from build123d import *

# Parameters (mm, degrees)
F1_DEPTH  = 38
F3_DEPTH  = 25
F4_DEPTH  = 38
F0_W      = 5
F0_H      = 28
F5_DEPTH  = 38
F6_DEPTH  = 34
F0_W_2    = 8.5
F0_H_2    = 23
F7_DEPTH  = 29
F8_DEPTH  = 24
F0_W_3    = 25
F9_DEPTH  = 19
F10_DEPTH = 10
F0_H_3    = 10
F11_DEPTH = 5
F12_DEPTH = 19


with BuildPart() as f1:
    # F0 (on Top) → F1 (new body)
    with BuildSketch(Plane.XY):
        Polygon((-33.5, -24), (-33.5, -14), (-33.5, -4), (-33.5, 19), (-38.5, 19), (-38.5, -24), align=None)
    extrude(amount=F1_DEPTH)

    # F2 (on face) → F3 (cut)
    with BuildSketch(Plane.YZ.offset(-33.5)):
        Polygon((-24, 19), (19, 38), (-24, 38), align=None)
    extrude(amount=-F3_DEPTH, mode=Mode.SUBTRACT)

    # F0 (on Top) → F4 (join)
    with BuildSketch(Plane.XY):
        Polygon((8.5, 19), (8.5, 24), (-38.5, 24), (-38.5, 19), (-33.5, 19), (-8.5, 19), (0, 19), align=None)
    extrude(amount=F4_DEPTH)



with BuildPart() as f5:
    # F0 (on Top) → F5 (new body)
    with BuildSketch(Plane.XY):
        with Locations((36, 10)):
            Rectangle(F0_W, F0_H)
    extrude(amount=F5_DEPTH)


with BuildPart() as f1_1:
    add(f1.part)

    add(f5.part)  # F6 merges F5
    # F0 (on Top) → F6 (join)
    with BuildSketch(Plane.XY):
        Polygon((8.5, -4), (33.5, -4), (33.5, 24), (8.5, 24), (8.5, 19), align=None)
    extrude(amount=F6_DEPTH)

    # F0 (on Top) → F7 (join)
    with BuildSketch(Plane.XY):
        with Locations((4.25, 7.5)):
            Rectangle(F0_W_2, F0_H_2)
    extrude(amount=F7_DEPTH)

    # F0 (on Top) → F8 (join)
    with BuildSketch(Plane.XY):
        with Locations((-4.25, 7.5)):
            Rectangle(F0_W_2, F0_H_2)
    extrude(amount=F8_DEPTH)

    # F0 (on Top) → F9 (join)
    with BuildSketch(Plane.XY):
        with Locations((-21, 7.5)):
            Rectangle(F0_W_3, F0_H_2)
    extrude(amount=F9_DEPTH)

    # F0 (on Top) → F10 (join)
    with BuildSketch(Plane.XY):
        Polygon((-8.5, -14), (33.5, -14), (33.5, -4), (8.5, -4), (0, -4), (-8.5, -4), (-33.5, -4), (-33.5, -14), align=None)
    extrude(amount=F10_DEPTH)

    # F0 (on Top) → F11 (join)
    with BuildSketch(Plane.XY):
        with Locations((-21, -19)):
            Rectangle(F0_W_3, F0_H_3)
    extrude(amount=F11_DEPTH)

    # F0 (on Top) → F12 (join)
    with BuildSketch(Plane.XY):
        Polygon((33.5, -24), (38.5, -24), (38.5, -4), (33.5, -4), (33.5, -14), align=None)
    extrude(amount=F12_DEPTH)


solid = f1_1.part
Work out the finished part from the listing and answer in its coordinate system (mm). A direction names the side the tool comes from. Give positions to 0.01 mm unless a question says otherwise; leave off trailing zeros. Loops run counter-clockwise (first coordinate to the right, second up) from the corner with the lowest first, then second, coordinate; pieces in that order, holes last. Notation, with made-up numbers: (7, 86.25) - (38, 86.25) arc R25 cw to (38, 125.25) - close; hole circle Ø11 at (39, 20.25). An arc over 180 degrees is marked (long way). Answer in a Markdown table with one row per item. Add a question column.
Q1. The part is cut by section A-A (y = -20). Determine the outline of the cut face in (x, z), and give its area (3 significant figures).
Q2. Determine the mould class of faces 4 (the flat face through (36, -24, 9)), 5 (the flat face through (0, -9, 10)) for opening direction X: released by +X, released by -X, zero draft, split by the parting line, or undercut.
Q3. The part is cut by section B-B (z = 6.5). Determine the outline of the cut face in (x, y).
Q4. Each of these flat-tipped pins is pushed along its axis until it touches: P1, Ø8, axis at x = -29, z = 26.5, coming from the -Y side; P2, Ø1.5, axis at x = 8.5, z = 12, coming from the -Y side; P3, Ø9.5, axis at x = -2.5, y = 7.5, coming from the +Z side. Where does it stop, or does it pass through?
Q5. Consider line 1 along X through (y, z) = (-17, 8); line 2 along X through (y, z) = (20, 36.5); line 3 along Y through (x, z) = (12, 23). Determine where each line is inside the solid, lowest interval first.
Q6. The part is cut by section D-D (z = 35.5). Determine the outline of the cut face in (x, y), and give its area (3 significant figures).
Q7. The part is cut by section C-C (x = -7). Determine the outline of the cut face in (y, z).
Q8. A tool of negligible diameter and unlimited length cuts with its end or side. For faces 1 (the flat face through (-33.5, -3, 21)), 2 (the flat face through (33.5, 10, 36)), 3 (the flat face through (-8.5, -19, 2)), from which of +Z, -Z, +X, -X, +Y, -Y can it reach the whole face along a straight path? Write none if from no direction.
Solution:
| question | item | result |
|---|---|---|
| 1 | outline | (-38.5, 0) - (-8.5, 0) - (-8.5, 5) - (-33.5, 5) - (-33.5, 20.77) - (-38.5, 20.77) - close; (33.5, 0) - (38.5, 0) - (38.5, 19) - (33.5, 19) - close |
| 1 | area | 324 mm² |
| 2 | face 4 | zero draft |
| 2 | face 5 | undercut |
| 3 | outline | (-38.5, -24) - (-33.5, -24) - (-33.5, -14) - (33.5, -14) - (33.5, -24) - (38.5, -24) - (38.5, 24) - (-38.5, 24) - close |
| 4 | P1 | stops at y = 19 |
| 4 | P2 | stops at y = -4 |
| 4 | P3 | stops at z = 29 |
| 5 | line 1 | x = -38.5 to -33.5, 33.5 to 38.5 |
| 5 | line 2 | x = -38.5 to 8.5, 33.5 to 38.5 |
| 5 | line 3 | y = -4 to 24 |
| 6 | outline | (-38.5, 13.34) - (-33.5, 13.34) - (-33.5, 19) - (8.5, 19) - (8.5, 24) - (-38.5, 24) - close; (33.5, -4) - (38.5, -4) - (38.5, 24) - (33.5, 24) - close |
| 6 | area | 403 mm² |
| 7 | outline | (-14, 0) - (24, 0) - (24, 38) - (19, 38) - (19, 24) - (-4, 24) - (-4, 10) - (-14, 10) - close |
| 8 | face 1 | +Z, -Y |
| 8 | face 2 | +Z, +Y, -Y |
| 8 | face 3 | +Z, -Z, -Y |
